Geometry: final body of the model. Coordinates: model frame, mm. Round coordinates to 2 decimals unless told otherwise and drop trailing zeros. Write each loop counter-clockwise with the first axis right and the second up, starting at its lowest first coordinate (ties: lowest second). Pieces come first, ordered by that corner, then holes. Notation, with made-up numbers: M 80,-27 L 118,-27 A31 cw 118,5 Z; hole C -2,-2.75 d8. An arc over 180 degrees is marked long. Use one line per item in the form item = value. Start each with the question number.
Item 1: Section query B-B (y = 0.7). Return loops of the section in (x, z), and give its area (3 significant figures).
Item 2: Section query A-A (x = 14). Return loops of the section in (y, z).
Item 3: Pin query (flat end, axial travel): pin 1 Ø2 at (x, z) = (14, 2.5) entering from +Y; pin 2 Ø1.6 at (x, z) = (7, 3) entering from +Y. Return the tip coordinate at first contact, or that it passes through.
Item 4: Ray query, probe 1 along X at (y, z) = (1.75, 6); probe 2 along X at (y, z) = (0.85, 6); probe 3 along Z at (x, y) = (17, 0.45). Return the intervals inside material, ascending.
Item 5: Section query C-C (z = 6). Return loops of the section in (x, y), and give its area (3 significant figures).
Item 6: Section query D-D (x = 3.5). Return loops of the section in (y, z).
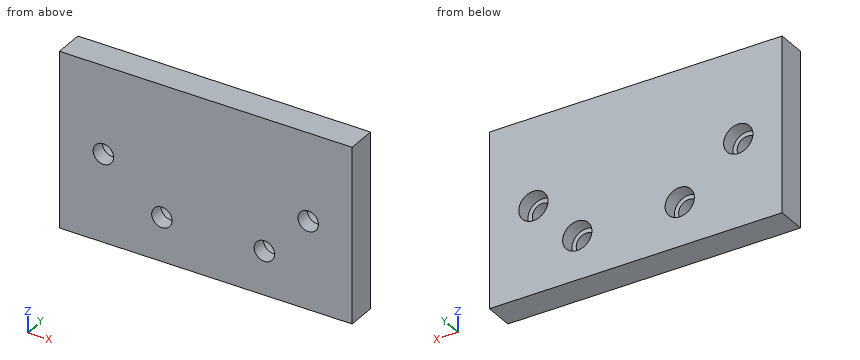
from build123d import *

# Parameters (mm, degrees)
SKETCH_1_W          = 20
SKETCH_1_H          = 12
SKETCH_1_R          = 0.7
EXTRUDE_1_DEPTH     = 2
CUT_EXTRUDE_START   = 2
SKETCH_1_3_R        = 1
CUT_EXTRUDE_1_DEPTH = 1


with BuildPart() as part:
    # 草图1 → 凸台-拉伸1 (new body)
    with BuildSketch(Plane(origin=(0, 0, 0), x_dir=(1, 0, 0), z_dir=(0, 1, 0))):
        with Locations((10, -6)):
            Rectangle(SKETCH_1_W, SKETCH_1_H)
        with Locations(Location((3, -6, 0), (0, 0, 270))):
            Circle(SKETCH_1_R, mode=Mode.SUBTRACT)
        with Locations(Location((7, -3, 0), (0, 0, 270))):
            Circle(SKETCH_1_R, mode=Mode.SUBTRACT)
        with Locations(Location((14, -3, 0), (0, 0, 270))):
            Circle(SKETCH_1_R, mode=Mode.SUBTRACT)
        with Locations(Location((17, -6, 0), (0, 0, 270))):
            Circle(SKETCH_1_R, mode=Mode.SUBTRACT)
    extrude(amount=EXTRUDE_1_DEPTH)

    # 草图1<3> → 切除-拉伸1 (cut)
    with BuildSketch(Plane(origin=(0, 0, 0), x_dir=(1, 0, 0), z_dir=(0, 1, 0)).offset(CUT_EXTRUDE_START)):
        with Locations(Location((3, -6, 0), (0, 0, 270))):
            Circle(SKETCH_1_3_R)
        with Locations(Location((7, -3, 0), (0, 0, 270))):
            Circle(SKETCH_1_3_R)
        with Locations(Location((14, -3, 0), (0, 0, 270))):
            Circle(SKETCH_1_3_R)
        with Locations(Location((17, -6, 0), (0, 0, 270))):
            Circle(SKETCH_1_3_R)
    extrude(amount=-CUT_EXTRUDE_1_DEPTH, mode=Mode.SUBTRACT)


solid = part.part
Working result:
q1.outline = M 0,0 L 20,0 L 20,12 L 0,12 Z; hole C 3,6 d1.4; hole C 7,3 d1.4; hole C 14,3 d1.4; hole C 17,6 d1.4
q1.area = 234 mm²
q2.outline = M 0,0 L 2,0 L 2,2 L 1,2 L 1,2.3 L 0,2.3 Z; M 0,3.7 L 1,3.7 L 1,4 L 2,4 L 2,12 L 0,12 Z
q3.pin_1 = 2
q3.pin_2 = 1
q4.probe_1 = 0 to 2, 4 to 16, 18 to 20
q4.probe_2 = 0 to 2.3, 3.7 to 16.3, 17.7 to 20
q4.probe_3 = 0 to 5.3, 6.7 to 12
q5.outline = M 0,0 L 2.3,0 L 2.3,1 L 2,1 L 2,2 L 0,2 Z; M 3.7,0 L 16.3,0 L 16.3,1 L 16,1 L 16,2 L 4,2 L 4,1 L 3.7,1 Z; M 17.7,0 L 20,0 L 20,2 L 18,2 L 18,1 L 17.7,1 Z
q5.area = 33.2 mm²
q6.outline = M 0,0 L 2,0 L 2,5.13 L 1,5.13 L 1,5.51 L 0,5.51 Z; M 0,6.49 L 1,6.49 L 1,6.87 L 2,6.87 L 2,12 L 0,12 Z
